from build123d import *

# Parameters (mm, degrees)
BOSS_EXTRUDE1_DEPTH            = 6
CHAMFER1_SIZE                  = 0.6
CBORE_FOR_M3_SHCS1_D           = 3.4
CBORE_FOR_M3_SHCS1_CBORE_D     = 6.5
CBORE_FOR_M3_SHCS1_CBORE_DEPTH = 3
DEBURS_SIZE                    = 0.2


with BuildPart() as part:
    # Sketch1 → Boss-Extrude1 (new body)
    with BuildSketch(Plane.XY):
        with BuildLine():
            Line((-5, -7.5), (-5, 7.5))
            ThreePointArc((-5, 7.5), (0, 12.5), (5, 7.5))
            Line((5, 7.5), (5, -7.5))
            ThreePointArc((5, -7.5), (0, -12.5), (-5, -7.5))
        make_face()
    extrude(amount=BOSS_EXTRUDE1_DEPTH)

    # Chamfer1
    chamfer1_edges = [part.edges().sort_by_distance(p)[0] for p in [
        (0, 12.5, 6),
        (-5, 0, 6),
        (0, -12.5, 6),
        (-5, 0, 0),
        (0, 12.5, 0),
        (5, 0, 0),
        (0, -12.5, 0),
        (5, 0, 6),
    ]]
    chamfer(chamfer1_edges, length=CHAMFER1_SIZE)

    # CBORE for M3 SHCS1 (through all)
    with Locations(Plane.XY.offset(6)):
        with Locations((0, 7.5), (0, -7.5)):
            CounterBoreHole(CBORE_FOR_M3_SHCS1_D / 2, CBORE_FOR_M3_SHCS1_CBORE_D / 2, CBORE_FOR_M3_SHCS1_CBORE_DEPTH)

    # Deburs
    deburs_edges = [part.edges().sort_by_distance(p)[0] for p in [
        (-3.25, -7.5, 6),
        (1.7, -7.5, 0),
        (1.7, -7.5, 3),
        (-3.25, 7.5, 6),
        (1.7, 7.5, 0),
        (1.7, 7.5, 3),
    ]]
    chamfer(deburs_edges, length=DEBURS_SIZE)


solid = part.part
Input: part model. Units: mm. Frame: model coordinates. A direction names the side the tool comes from. Coordinates: 2 decimals unless noted, no trailing zeros. Loops run counter-clockwise (first coordinate to the right, second up) from the corner with the lowest first, then second, coordinate; pieces in that order, holes last. Notation, with made-up numbers: (29.5, -22.75) -> (65.5, -22.75) arc R22 cw to (65.5, 2.25) -> close; hole circle Ø6 at (43.5, -9.75). An arc over 180 degrees is marked (long way). Write each question's results on one line, items separated by ' | '. Start each with the question number.
Q1. Section B-B, the plane x = 0. State how many separate pieces and enclosed holes the cut face has, plus the area to 3 significant figures.
Q2. Reachability of faces 1 (the cylindrical face through (-0.423, -4.278, 4.42)), 2 (the cylindrical face through (0.37, -9.16, 1.48)) from +Z, -Z, +X, -X, +Y, -Y: full face, straight path, thin tool, end or side. Return the list, or none.
Q3. Ray query, line 1 (Y direction, x = 0, z = 1.2); line 2 (Y direction, x = 0, z = 3.7); line 3 (X direction, y = 6.75, z = 4.75). Return the intervals inside material, ascending. Write a range as from..to.
Q4. Pin query (flat end, axial travel): pin 1 (1 mm diameter, centred on y = -9.5, z = 3.5, fed in from +X); pin 2 (5 mm diameter, centred on x = 0, y = 7.5, fed in from +Z); pin 3 (1.5 mm diameter, centred on x = 3.5, z = 4.5, fed in from +Y). Return the tip coordinate at first contact, or that it passes through.
Q5. Pull-direction query (X, two-part tool) for faces 3 (the cylindrical face through (-0.1, 12.5, 3)), 4 (the flat face through (-5, 0, 3)), 5 (the flat face through (5, 0, 3)), 6 (the cylindrical face through (1.75, 10.24, 4.42)); classes: released by +X, released by -X, zero draft, split by the parting line, or undercut.
Q6. Section A-A, the plane z = 4. Return the cut outline in (x, y).
Found:
1) separate pieces: 3 | enclosed holes: 0 | area: 89.6 mm2
2) face 1: +Z | face 2: +Z, -Z
3) line 1: -12.5..-9.2, -5.8..5.8, 9.2..12.5 | line 2: -12.5..-10.75, -4.25..4.25, 10.75..12.5 | line 3: -5..-3.16, 3.16..5
4) pin 1: x = 4.77 | pin 2: z = 3 | pin 3: y = 11.68
5) face 3: split by the parting line | face 4: released by -X | face 5: released by +X | face 6: undercut
6) outline: (-5, -7.5) arc R5 ccw to (5, -7.5) -> (5, 7.5) arc R5 ccw to (-5, 7.5) -> close; hole circle Ø6.5 at (0, -7.5); hole circle Ø6.5 at (0, 7.5)
